Read the model definition and answer for the solid it produces. Units are mm, in the model's axes. Face numbers are marked on the shaded views. A direction names the side the tool comes from. Coordinates: 2 decimals unless noted, no trailing zeros. Write each loop counter-clockwise with the first axis right and the second up, starting at its lowest first coordinate (ties: lowest second). Pieces come first, ordered by that corner, then holes. Notation, with made-up numbers: (36.25, -34) -> (49.25, -34) arc R14 cw to (49.25, -14) -> close; hole circle Ø4 at (-34, -38.5). An arc over 180 degrees is marked (long way). Answer in a Markdown table with one row per item. Add a question column.
Item 1: Which of the six approach directions +Z, -Z, +X, -X, +Y, -Y give full straight-line access (tool end or side, diameter ignored) to the marked faces 1, 2, 3, 4 and 5?
Item 2: Given pin 1 Ø8 at (x, z) = (17, 15.5) entering from +Y; pin 2 Ø9 at (y, z) = (12.5, 10) entering from -X; pin 3 Ø5.5 at (y, z) = (9, 6) entering from -X; pin 4 Ø2.5 at (x, y) = (-78, 40) entering from -Z, each flat-ended and moving along its own axis, determine where each tip first touches the part or whether it passes through.
Item 3: For a pull along X with two mould halves and no side action, classify the marked faces 6, 7, 8 and 9 as +X half, -X half, draft (parallel to the pull), parting line (faces both ways), or undercut.
Item 4: Section A-A on x = -67 is taken. Write down the section's boundary in (y, z), then the cut area to 3 significant figures.
Item 5: Straight lines are drawn through the part: line 1 (X direction, y = 16, z = 8.25); line 2 (X direction, y = 36, z = 2.25) (3 decimals); line 3 (Y direction, x = -37, z = 12.5). For each, find the intervals that lie inside material, in ascending order. Write a range as from..to.
Item 6: Section D-D on x = 47 is taken. Write down the section's boundary in (y, z).
Item 7: Section B-B on x = 16 is taken. Write down the section's boundary in (y, z).
Item 8: Section C-C on z = 4 is taken. Count the separate pieces of the cut face and the enclosed holes in it, then the cut area to 3 significant figures.
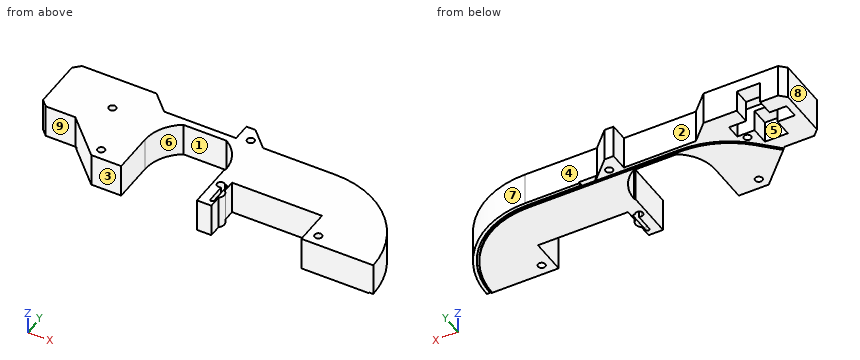
```python
from build123d import *

# Parameters (mm, degrees)
SKETCH_R        = 2
PAD_DEPTH       = 18.5
POCKET_DEPTH    = 1.25
POCKET001_DEPTH = 12
SKETCH005_W     = 32
SKETCH005_H     = 8
POCKET002_DEPTH = 15
POCKET003_DEPTH = 0.5


with BuildPart() as part:
    # Sketch → Pad (new body)
    with BuildSketch(Plane.XY):
        with BuildLine():
            Line((0, 20), (50, 20))
            Line((50, 20), (50, 0))
            Line((50, 0), (90, 0))
            ThreePointArc((90, 0), (75.3553391883, 35.3553389303), (40.0000003648, 50))
            Line((0, 50), (40.0000003648, 50))
            Line((-10, 60), (0, 50))
            Line((-15, 60), (-10, 60))
            Line((-15, 50), (-15, 60))
            Line((-55, 50), (-15, 50))
            Line((-65, 60), (-55, 50))
            Line((-106.4644660941, 60), (-65, 60))
            Line((-110, 56.4644660941), (-106.4644660941, 60))
            Line((-110, 28.5355339059), (-110, 56.4644660941))
            Line((-106.4644660941, 25), (-110, 28.5355339059))
            Line((-90, 25), (-106.4644660941, 25))
            Line((-69.14, 4.14), (-90, 25))
            Line((-52.5, 4.14), (-69.14, 4.14))
            Line((-52.5, 4.14), (-52.5, 27.0000073596))
            ThreePointArc((-42.0519707932, 46), (-49.7157196548, 37.8416049777), (-52.5, 27.0000073596))
            Line((-42.0519707932, 46), (-17.9480292068, 46))
            ThreePointArc((-7.5, 27), (-10.2842785721, 37.8416017533), (-17.9480292068, 46))
            Line((-7.5, 27), (-8, 26.5))
            Line((-8, 26.5), (-8, 0))
            Line((0, 0), (-8, 0))
            Line((0, 0), (0, 7.1277186767))
            ThreePointArc((0, 7.1277186767), (1.5, 10), (0, 12.8722813233))
            Line((0, 20), (0, 12.8722813233))
        make_face()
        with Locations((56, 6)):
            Circle(SKETCH_R, mode=Mode.SUBTRACT)
        with Locations((-8, 52)):
            Circle(SKETCH_R, mode=Mode.SUBTRACT)
        with Locations((-67, 10)):
            Circle(SKETCH_R, mode=Mode.SUBTRACT)
        with Locations((-78, 40)):
            Circle(SKETCH_R, mode=Mode.SUBTRACT)
        with BuildLine():
            ThreePointArc((-2.2083333333, 16.8887803753), (-5.6996412833, 17.0541439694), (-3.9999998699, 14))
            Line((-3.9999998699, 14), (-2.75, 14))
            Line((-2.75, 14), (-2.75, 4))
            ThreePointArc((-2.75, 4), (-1.75, 3), (-0.75, 4))
            Line((-0.75, 16), (-0.75, 4))
            ThreePointArc((-0.75, 16), (-1.2295835001, 16.8539125638), (-2.2083333333, 16.8887803753))
        make_face(mode=Mode.SUBTRACT)
    extrude(amount=PAD_DEPTH)

    # SubtractivePipe: sweep along a path in Sketch001
    with BuildLine(Plane.XY.offset(18.5)) as subtractivepipe_path:
        Line((-72.9307178569, 0), (-58.9653554732, 13.9653623837))
        ThreePointArc((-58.9653554732, 13.9653623837), (-52.5579955482, 18.2466216954), (-45.0000000351, 19.75))
        Line((-45.0000000351, 19.75), (39.9999998281, 19.75))
        ThreePointArc((39.9999998281, 19.75), (53.9653588677, 13.9653589892), (59.75, 0))
    # Sketch002 (on DatumPlane) → SubtractivePipe (sweep, cut)
    with BuildSketch(Plane(origin=(-32.5, -32.5, 0), x_dir=(0.7071067812, -0.7071067812, 0), z_dir=(-0.7071067812, -0.7071067812, 0))):
        Polygon((-80, -18.75), (-70, -18.75), (-70, -0.25), (-78.75, -0.25), (-78.75, 1.25), (-80, 1.25), align=None)
    sweep(path=subtractivepipe_path.line, mode=Mode.SUBTRACT)

    # Sketch003 → Pocket (cut)
    with BuildSketch(Plane.XY):
        Polygon((0, 50), (2, 48), (10, 48), (10, 50), align=None)
    extrude(amount=POCKET_DEPTH, mode=Mode.SUBTRACT)

    # Sketch004 → Pocket001 (cut)
    with BuildSketch(Plane.XY):
        Polygon((-96.5, 60), (-96.5, 50.5), (-96.375, 50.5), (-96.375, 33), (-83.625, 33), (-83.625, 50.5), (-83.5, 50.5), (-83.5, 60), align=None)
    extrude(amount=POCKET001_DEPTH, mode=Mode.SUBTRACT)

    # Sketch005 → Pocket002 (cut)
    with BuildSketch(Plane.XY):
        with Locations((-90, 47)):
            Rectangle(SKETCH005_W, SKETCH005_H)
    extrude(amount=POCKET002_DEPTH, mode=Mode.SUBTRACT)

    # Sketch006 → Pocket003 (cut)
    with BuildSketch(Plane.XY):
        with BuildLine():
            ThreePointArc((87.7395276474, -1), (74.1160702602, 33.4089247058), (40, 47.75))
            Line((40, 47.75), (9.5, 47.75))
            Line((9.5, 47.75), (9.5, 50.25))
            Line((9.5, 50.25), (39.9999271709, 50.25))
            ThreePointArc((90.2400487659, -1), (75.8839019692, 35.1768116729), (39.9999271709, 50.2499999999))
            Line((87.7395276474, -1), (90.2400487659, -1))
        make_face()
    extrude(amount=POCKET003_DEPTH, mode=Mode.SUBTRACT)


solid = part.part
```
Results below:
| question | item | result |
|---|---|---|
| 1 | face 1 | +Z, -Z, -Y |
| 1 | face 2 | +Z, -Z, +Y |
| 1 | face 3 | +Z, -Z, -X, -Y |
| 1 | face 4 | +Z, -Z, +X, +Y |
| 1 | face 5 | -Z, +Y |
| 2 | pin 1 | stops at y = 50 |
| 2 | pin 2 | stops at x = -82 |
| 2 | pin 3 | stops at x = -76.75 |
| 2 | pin 4 | passes through |
| 3 | face 6 | undercut |
| 3 | face 7 | +X half |
| 3 | face 8 | -X half |
| 3 | face 9 | draft |
| 4 | outline | (4.14, 0) -> (8, 0) -> (8, 18.5) -> (4.14, 18.5) -> close; (12, 0) -> (41.45, 0) -> (41.45, 1.25) -> (42.86, 1.25) -> (42.86, 0) -> (60, 0) -> (60, 18.5) -> (12, 18.5) -> close |
| 4 | area | 958 mm2 |
| 5 | line 1 | x = -81..-52.5, -8..-6, -0.75..0, 50..87.37 |
| 5 | line 2 | x = -110..-96.375, -83.625..-50.622, -9.378..74.699 |
| 5 | line 3 | y = 46..50 |
| 6 | outline | (20, 0) -> (46.41, 0) -> (46.41, 1.25) -> (47.67, 1.25) -> (47.67, 0.5) -> (49.51, 0.5) -> (49.51, 18.5) -> (20, 18.5) -> close |
| 7 | outline | (20, 0) -> (46.93, 0) -> (46.93, 1.25) -> (48.18, 1.25) -> (48.18, 0.5) -> (50, 0.5) -> (50, 18.5) -> (20, 18.5) -> close |
| 8 | separate pieces | 1 |
| 8 | enclosed holes | 5 |
| 8 | area | 5,660 mm2 |
